Read the model definition and answer for the solid it produces. Units are mm, in the model's axes. Give positions to 0.01 mm unless a question says otherwise; leave off trailing zeros. Loops run counter-clockwise (first coordinate to the right, second up) from the corner with the lowest first, then second, coordinate; pieces in that order, holes last.
(1) Determine the mould class of faces 1 (the face through (3, -8, 1)), 2 (the face through (2.898, -10.696, 7.858)), 3 (the face through (18.792, -20.154, 0.507)), 4 (the face through (0, -11.2, 0.5)) for opening direction X: pulls with the +X half, pulls with the -X half, needs draft (parallel to the pull), parting line crosses it, or undercut.
(2) Find section B-B, the plane x = 10.95. Write down the section's boundary in (y, z), then the cut area to 3 significant figures.
(3) Find section D-D, the plane z = 3. Write down the section's boundary in (x, y), then the cut area to 3 significant figures.
(4) Find section A-A, the plane y = -2.56. Write down the section's boundary in (x, z).
(5) Each of these flat-tipped pins is pushed along its axis until it touches: P1, Ø8, axis at y = -7, z = 7, coming from the -X side; P2, Ø2.5, axis at x = 17.36, y = -19.56, coming from the -Z side; P3, Ø1, axis at y = -9, z = 8.5, coming from the +X side; P4, Ø6, axis at x = 8.5, z = 13.5, coming from the +Y side. Where does it stop, or does it pass through?
(6) Straight lines are drawn through the part: probe 1 along Y at (x, z) = (17.36, 0.45); probe 2 along Y at (x, z) = (4.76, 0.75); probe 3 along Z at (x, y) = (1, -2). For each, find the intervals that lie inside material, in ascending order.
(7) Find section C-C, the plane y = -11.05. Write down the section's boundary in (x, z), then the cut area to 3 significant figures.
```python
from build123d import *

# Parameters (mm, degrees)
SKETCH1_W      = 19.9
SKETCH1_H      = 22.1
EXTRUDE1_DEPTH = 1
SKETCH2_R      = 1.55
EXTRUDE2_DEPTH = 1
SKETCH3_R      = 8.06
EXTRUDE3_DEPTH = 14.41
FILLET1_R      = 0.5


with BuildPart() as part:
    # Sketch1 → Extrude1 (new body)
    with BuildSketch(Plane.XY):
        with Locations((9.95, -11.05)):
            Rectangle(SKETCH1_W, SKETCH1_H)
    extrude(amount=EXTRUDE1_DEPTH)

    # Sketch2 → Extrude2 (cut)
    with BuildSketch(Plane.XY.offset(1)):
        with Locations((4.76, -2.56)):
            Circle(SKETCH2_R)
        with Locations((17.36, -19.56)):
            Circle(SKETCH2_R)
    extrude(amount=-EXTRUDE2_DEPTH, mode=Mode.SUBTRACT)

    # Sketch3 → Extrude3 (add)
    with BuildSketch(Plane.XY.offset(1)):
        with Locations((10.95, -11.05)):
            Circle(SKETCH3_R)
    extrude(amount=EXTRUDE3_DEPTH)

    # Fillet1
    fillet1_edges = [part.edges().sort_by_distance(p)[0] for p in [
        (2.89, -11.05, 15.41),
    ]]
    fillet(fillet1_edges, radius=FILLET1_R)


solid = part.part
```
Entries:
1. face 1: needs draft
1. face 2: parting line crosses it
1. face 3: undercut
1. face 4: pulls with the -X half
2. outline: (-22.1, 0) - (0, 0) - (0, 1) - (-2.99, 1) - (-2.99, 14.91) arc R0.5 ccw to (-3.49, 15.41) - (-18.61, 15.41) arc R0.5 ccw to (-19.11, 14.91) - (-19.11, 1) - (-22.1, 1) - close
2. area: 254 mm2
3. outline: circle Ø16.12 at (10.95, -11.05)
3. area: 204 mm2
4. outline: (0, 0) - (3.21, 0) - (3.21, 1) - (0, 1) - close; (6.31, 0) - (19.9, 0) - (19.9, 1) - (6.31, 1) - close
5. P1: stops at x = 2.89
5. P2: passes through
5. P3: stops at x = 18.86
5. P4: stops at y = -2.99
6. probe 1: y = -22.1 to -21.11, -18.01 to 0
6. probe 2: y = -22.1 to -4.11, -1.01 to 0
6. probe 3: z = 0 to 1
7. outline: (0, 0) - (19.9, 0) - (19.9, 1) - (19.01, 1) - (19.01, 14.91) arc R0.5 ccw to (18.51, 15.41) - (3.39, 15.41) arc R0.5 ccw to (2.89, 14.91) - (2.89, 1) - (0, 1) - close
7. area: 252 mm2
